from build123d import *

# Parameters (mm, degrees)
EXTRUDE_THIN1_DEPTH = 25.4
SKETCH2_R           = 3.9751
SKETCH2_R_2         = 1.3208
CUT_EXTRUDE1_DEPTH  = 48.307499936
SKETCH3_R           = 2.4892
CUT_EXTRUDE2_DEPTH  = 2.5875


with BuildPart() as part:
    # Sketch1 → Extrude-Thin1 (new body)
    with BuildSketch(Plane.XY):
        Polygon((0, 0), (0, 25.4), (45.719999936, 25.4), (45.719999936, 78.74), (47.307499936, 78.74), (47.307499936, 23.8125), (1.5875, 23.8125), (1.5875, 0), align=None)
    extrude(amount=EXTRUDE_THIN1_DEPTH)

    # Sketch2 → Cut-Extrude1 (cut, through all)
    with BuildSketch(Plane(origin=(47.307499936, 0, 0), x_dir=(0, 0, -1), z_dir=(1, 0, 0))):
        with Locations((-12.7, 66.04)):
            Circle(SKETCH2_R)
        with Locations((-18.796293344, 61.771329445)):
            Circle(SKETCH2_R_2)
        with Locations((-6.603706656, 70.308670555)):
            Circle(SKETCH2_R_2)
    extrude(amount=-CUT_EXTRUDE1_DEPTH, mode=Mode.SUBTRACT)

    # Sketch3 → Cut-Extrude2 (cut, through all)
    with BuildSketch(Plane(origin=(1.5875, 0, 0), x_dir=(0, 0, -1), z_dir=(1, 0, 0))):
        with Locations((-19.05, 12.7)):
            Circle(SKETCH3_R)
        with Locations((-6.35, 12.7)):
            Circle(SKETCH3_R)
    extrude(amount=-CUT_EXTRUDE2_DEPTH, mode=Mode.SUBTRACT)


solid = part.part
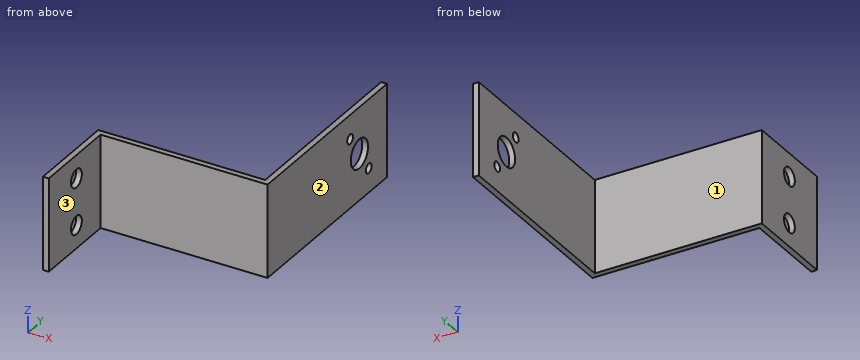
Can you work these out from the model? Positions are in its coordinate system, mm. Face numbers are marked on the shaded views. A direction names the side the tool comes from. Round coordinates to 2 decimals unless told otherwise and drop trailing zeros. Order: outer loops, then holes, each group sorted by start corner. A loop starts at its lowest first (then second) coordinate and runs counter-clockwise, first axis right, second up. Notation, with made-up numbers: (-23.75, 28.25) - (12.25, 28.25) arc R7 ccw to (12.25, 32.25) - close; hole circle Ø11 at (8, 28.5). An arc over 180 degrees is marked (long way). Answer in a Markdown table with one row per item.
(1) Suppose I cut it at B-B, the plane z = 19.05. Please give me the cut outline in (x, y).
From the geometry:
| item | result |
|---|---|
| outline | (0, 0) - (1.59, 0) - (1.59, 10.21) - (0, 10.21) - close; (0, 15.19) - (1.59, 15.19) - (1.59, 23.81) - (47.31, 23.81) - (47.31, 60.48) - (45.72, 60.48) - (45.72, 25.4) - (0, 25.4) - close; (45.72, 63.07) - (47.31, 63.07) - (47.31, 78.74) - (45.72, 78.74) - close |
(2) Which directions (+Z, -Z, +X, -X, +Y, -Y) give clear straight access to the entire face, cutting with the end or side of a thin tool? Please do the marked faces 1, 2 and 3.
From the geometry:
| item | result |
|---|---|
| face 1 | +Z, -Z, -X, +Y |
| face 2 | +Z, -Z, +X, +Y, -Y |
| face 3 | +Z, -Z, +X, -Y |
(3) Suppose I cut it at C-C, the plane z = 12.5. Please give me the cut outline in (x, y), plus the area to 3 significant figures.
From the geometry:
| item | result |
|---|---|
| outline | (0, 0) - (1.59, 0) - (1.59, 23.81) - (47.31, 23.81) - (47.31, 62.07) - (45.72, 62.07) - (45.72, 25.4) - (0, 25.4) - close; (45.72, 70.01) - (47.31, 70.01) - (47.31, 78.74) - (45.72, 78.74) - close |
| area | 185 mm2 |
(4) Please list where these lines run through material, in increasing order: L1, parallel to X at y = 35, z = 8.5; L2, parallel to Y at x = 0.65, z = 19.05; L3, parallel to Y at x = 41.5, z = 5. Write a range as from..to.
From the geometry:
| item | result |
|---|---|
| L1 | x = 45.72..47.31 |
| L2 | y = 0..10.21, 15.19..25.4 |
| L3 | y = 23.81..25.4 |
(5) For P1, Ø12.5, axis at y = 44, z = 13.5, coming from the -X side; P2, Ø7.5, axis at x = 28.5, z = 11.5, coming from the +Y side; P3, Ø4, axis at x = 39, z = 10, coming from the -Y side, each with a flat end and sliding along its axis, tell me the tip position at first contact or that it passes through.
From the geometry:
| item | result |
|---|---|
| P1 | stops at x = 45.72 |
| P2 | stops at y = 25.4 |
| P3 | stops at y = 23.81 |
(6) Suppose I cut it at D-D, the plane y = 55.5. Please give me the cut outline in (x, z), plus the area to 3 significant figures.
From the geometry:
| item | result |
|---|---|
| outline | (45.72, 0) - (47.31, 0) - (47.31, 25.4) - (45.72, 25.4) - close |
| area | 40.3 mm2 |
(7) Suppose I cut it at A-A, the plane y = 66.04. Please give me the cut outline in (x, z), plus the area to 3 significant figures.
From the geometry:
| item | result |
|---|---|
| outline | (45.72, 0) - (47.31, 0) - (47.31, 8.72) - (45.72, 8.72) - close; (45.72, 16.68) - (47.31, 16.68) - (47.31, 25.4) - (45.72, 25.4) - close |
| area | 27.7 mm2 |
